Model file for the job. Use its own axes, mm. A direction names the side the tool comes from. Coordinates: 2 decimals unless noted, no trailing zeros. Write each loop counter-clockwise with the first axis right and the second up, starting at its lowest first coordinate (ties: lowest second). Pieces come first, ordered by that corner, then holes. Notation, with made-up numbers: M 44,37 L 66,37 A15 cw 66,60 Z; hole C 60,-19 d7. An arc over 180 degrees is marked long. One line per question, with ' | ' between items. Start each with the question number.
(1) Flat gauge pins, fed straight in: pin 1 Ø1 at (y, z) = (-1.5, -4) entering from -X; pin 2 Ø4 at (y, z) = (4, -33.5) entering from +X; pin 3 Ø11 at (x, y) = (45.5, 7) entering from +Z. Where does each tip first touch, or does it go through?
(2) Cut at A-A (y = 8). Write the cut outline in (x, z).
(3) Cut at D-D (x = 8.5). Write the cut outline in (y, z) (1 decimal), plus the area to 3 significant figures.
(4) Cut at B-B (x = 37). Write the cut outline in (y, z) (1 decimal).
(5) Two-plate mould, pull along X, no slides. Class faces 4 (the face through (1, -1, -8.588)), 5 (the face through (0, 6, -35)), 6 (the face through (42, 6, -35)): +X half, -X half, draft (parallel to the pull), parting line (faces both ways), or undercut.
(6) Tool access for faces 1 (the face through (-5, -1, -28)), 2 (the face through (41, -1, -8.588)), 3 (the face through (47, 10, -6)): list every direction of +Z, -Z, +X, -X, +Y, -Y with a clear straight run to the whole face (end or side of a thin tool).
(7) Cut at C-C (y = 3.75). Write the cut outline in (x, z), plus the area to 3 significant figures.
(8) Wall check: probe 1 along X at (y, z) = (8, -34.65); probe 2 along Z at (x, y) = (48.5, 17); probe 3 along Z at (x, y) = (37, 11). Give the ranges that are in metal, low to high.
from build123d import *

# Parameters (mm, degrees)
SKETCH1_W                    = 42
SKETCH1_H                    = 36
BASE_FLANGE1_DEPTH           = 2
SKETCH6_W                    = 10
SKETCH6_H                    = 24
TAB1_DEPTH                   = 2
SKETCH9_W                    = 10
SKETCH9_H                    = 24
TAB2_DEPTH                   = 2
EDGE_FLANGE1_STRIP_W         = 11.175
EDGE_FLANGE1_STRIP_H         = 2
EDGE_FLANGE1_STRIP_CUT_DEPTH = 42
EDGE_FLANGE1_DEPTH           = 42
EDGE_FLANGE2_START           = -10
EDGE_FLANGE2_DEPTH           = 11
EDGE_FLANGE2_2_DEPTH         = 1
EDGE_FLANGE2_3_DEPTH         = 10
EDGE_FLANGE3_START           = 41
EDGE_FLANGE3_DEPTH           = 11
EDGE_FLANGE3_2_DEPTH         = 1
EDGE_FLANGE3_START_2         = 42
EDGE_FLANGE3_3_DEPTH         = 10
SKETCH21_W                   = 1
SKETCH21_H                   = 4
CUT_EXTRUDE1_DEPTH           = 10
SKETCH22_W                   = 1
SKETCH22_H                   = 4
CUT_EXTRUDE2_DEPTH           = 2
SKETCH23_W                   = 1.5
SKETCH23_H                   = 8.5875
CUT_EXTRUDE3_DEPTH           = 2
SKETCH24_W                   = 1.5
SKETCH24_H                   = 8.5875
CUT_EXTRUDE4_DEPTH           = 2
CUT_EXTRUDE5_REACH           = 67.757
SKETCH26_R                   = 2.5


# Read off the part's stored shape, not the designer's step: Edge-Flange2, Edge-Flange3
# Sheet-metal steps are written as plain solids
with BuildPart() as part:
    # Sketch1 → Base-Flange1 (new body)
    with BuildSketch(Plane(origin=(0, 0, 0), x_dir=(1, 0, 0), z_dir=(0, 1, 0))):
        with Locations((21, 18)):
            Rectangle(SKETCH1_W, SKETCH1_H)
    extrude(amount=-BASE_FLANGE1_DEPTH)

    # Sketch6 → Tab1 (add)
    with BuildSketch(Plane(origin=(0, 0, 0), x_dir=(1, 0, 0), z_dir=(0, 1, 0))):
        with Locations((47, 16)):
            Rectangle(SKETCH6_W, SKETCH6_H)
    extrude(amount=-TAB1_DEPTH)

    # Sketch9 → Tab2 (add)
    with BuildSketch(Plane(origin=(0, 0, 0), x_dir=(1, 0, 0), z_dir=(0, 1, 0))):
        with Locations((-5, 16)):
            Rectangle(SKETCH9_W, SKETCH9_H)
    extrude(amount=-TAB2_DEPTH)

    # Edge-Flange1 strip (across the edge) → Edge-Flange1 strip cut (cut)
    with BuildSketch(Plane(origin=(42, 0, -36), x_dir=(0, 0, 1), z_dir=(-1, 0, 0))):
        with Locations((-2, -1)):
            Rectangle(EDGE_FLANGE1_STRIP_W, EDGE_FLANGE1_STRIP_H)
    extrude(amount=EDGE_FLANGE1_STRIP_CUT_DEPTH, mode=Mode.SUBTRACT)

    # Edge-Flange1 section (across the edge) → Edge-Flange1 (add)
    with BuildSketch(Plane(origin=(42, 0, -36), x_dir=(0, 0, 1), z_dir=(-1, 0, 0))):
        with BuildLine():
            Line((0, 1.5875), (0, 18))
            Line((0, 18), (2, 18))
            Line((2, 18), (2, 1.5875))
            ThreePointArc((2, 1.5875), (2.464967985, 0.464967985), (3.5875, 0))
            Line((3.5875, 0), (3.5875, -2))
            ThreePointArc((3.5875, -2), (1.050754422, -0.949245578), (0, 1.5875))
        make_face()
    extrude(amount=EDGE_FLANGE1_DEPTH)

    # Edge-Flange2 outline → Edge-Flange2 (cut)
    with BuildSketch(Plane.YZ.offset(EDGE_FLANGE2_START)):
        with BuildLine():
            ThreePointArc((-2, -7.5875), (-1.45924519, -5.693430307), (0, -4.370358411))
            Line((0, -4.370358411), (0, -4))
            Line((0, -4), (-2, -4))
            Line((-2, -4), (-2, -7.5875))
        make_face()
    extrude(amount=EDGE_FLANGE2_DEPTH, mode=Mode.SUBTRACT)

    # Edge-Flange2 2 outline → Edge-Flange2 2 (cut)
    with BuildSketch(Plane.YZ):
        with BuildLine():
            Line((0, -8.5875), (0, -4.370358411))
            ThreePointArc((0, -4.370358411), (-1.45924519, -5.693430307), (-2, -7.5875))
            Line((-2, -7.5875), (-2, -8.5875))
            Line((-2, -8.5875), (0, -8.5875))
        make_face()
    extrude(amount=EDGE_FLANGE2_2_DEPTH, mode=Mode.SUBTRACT)

    # Edge-Flange2 3 outline → Edge-Flange2 3 (add)
    with BuildSketch(Plane.YZ.offset(EDGE_FLANGE2_START)):
        with BuildLine():
            Line((18, -4), (1.5875, -4))
            ThreePointArc((1.5875, -4), (0.77243534, -4.093816292), (0, -4.370358411))
            Line((0, -4.370358411), (0, -7.5875))
            ThreePointArc((0, -7.5875), (0.464967985, -6.464967985), (1.5875, -6))
            Line((1.5875, -6), (18, -6))
            Line((18, -6), (18, -4))
        make_face()
    extrude(amount=EDGE_FLANGE2_3_DEPTH)

    # Edge-Flange3 outline → Edge-Flange3 (cut)
    with BuildSketch(Plane.YZ.offset(EDGE_FLANGE3_START)):
        with BuildLine():
            ThreePointArc((-2, -7.5875), (-1.45924519, -5.693430307), (0, -4.370358411))
            Line((0, -4.370358411), (0, -4))
            Line((0, -4), (-2, -4))
            Line((-2, -4), (-2, -7.5875))
        make_face()
    extrude(amount=EDGE_FLANGE3_DEPTH, mode=Mode.SUBTRACT)

    # Edge-Flange3 2 outline → Edge-Flange3 2 (cut)
    with BuildSketch(Plane.YZ.offset(EDGE_FLANGE3_START)):
        with BuildLine():
            Line((0, -8.5875), (0, -4.370358411))
            ThreePointArc((0, -4.370358411), (-1.45924519, -5.693430307), (-2, -7.5875))
            Line((-2, -7.5875), (-2, -8.5875))
            Line((-2, -8.5875), (0, -8.5875))
        make_face()
    extrude(amount=EDGE_FLANGE3_2_DEPTH, mode=Mode.SUBTRACT)

    # Edge-Flange3 3 outline → Edge-Flange3 3 (add)
    with BuildSketch(Plane.YZ.offset(EDGE_FLANGE3_START_2)):
        with BuildLine():
            Line((18, -6), (18, -4))
            Line((18, -4), (1.5875, -4))
            ThreePointArc((1.5875, -4), (0.77243534, -4.093816292), (0, -4.370358411))
            Line((0, -4.370358411), (0, -7.5875))
            ThreePointArc((0, -7.5875), (0.464967985, -6.464967985), (1.5875, -6))
            Line((1.5875, -6), (18, -6))
        make_face()
    extrude(amount=EDGE_FLANGE3_3_DEPTH)

    # Sketch21 → Cut-Extrude1 (cut)
    with BuildSketch(Plane(origin=(0, 0, 0), x_dir=(1, 0, 0), z_dir=(0, 1, 0))):
        with Locations((0.5, 2)):
            Rectangle(SKETCH21_W, SKETCH21_H)
    extrude(amount=-CUT_EXTRUDE1_DEPTH, mode=Mode.SUBTRACT)

    # Sketch22 → Cut-Extrude2 (cut)
    with BuildSketch(Plane(origin=(0, 0, 0), x_dir=(1, 0, 0), z_dir=(0, 1, 0))):
        with Locations((41.5, 2)):
            Rectangle(SKETCH22_W, SKETCH22_H)
    extrude(amount=-CUT_EXTRUDE2_DEPTH, mode=Mode.SUBTRACT)

    # Sketch23 → Cut-Extrude3 (cut)
    with BuildSketch(Plane(origin=(0, 0, 0), x_dir=(1, 0, 0), z_dir=(0, 1, 0))):
        with Locations((1.75, 4.29375)):
            Rectangle(SKETCH23_W, SKETCH23_H)
    extrude(amount=-CUT_EXTRUDE3_DEPTH, mode=Mode.SUBTRACT)

    # Sketch24 → Cut-Extrude4 (cut)
    with BuildSketch(Plane(origin=(0, 0, 0), x_dir=(1, 0, 0), z_dir=(0, 1, 0))):
        with Locations((40.25, 4.29375)):
            Rectangle(SKETCH24_W, SKETCH24_H)
    extrude(amount=-CUT_EXTRUDE4_DEPTH, mode=Mode.SUBTRACT)

    # Sketch26 → Cut-Extrude5 (cut, up to next)
    with BuildSketch(Plane(origin=(0, 0, -36), x_dir=(-1, 0, 0), z_dir=(0, 0, -1)), mode=Mode.PRIVATE) as cut_extrude5_sk1:
        with Locations(Location((-37, 8, 0), (0, 0, 90))):
            Circle(SKETCH26_R)
    cut_extrude5_tool1 = extrude(cut_extrude5_sk1.sketch, amount=-CUT_EXTRUDE5_REACH, mode=Mode.PRIVATE) & part.part
    add(cut_extrude5_tool1.solids().sort_by_distance((37, 8, -36))[0], mode=Mode.SUBTRACT)


solid = part.part
Filled in:
1) pin 1: x = 2.5 | pin 2: x = 42 | pin 3: z = -4
2) outline: M -10,-6 L 0,-6 L 0,-4 L -10,-4 Z; M 0,-36 L 34.5,-36 L 34.5,-34 L 0,-34 Z; M 39.5,-36 L 42,-36 L 42,-34 L 39.5,-34 Z; M 42,-6 L 52,-6 L 52,-4 L 42,-4 Z
3) outline: M -2,-32.4 A3.6 ccw 1.6,-36 L 18,-36 L 18,-34 L 1.6,-34 A1.6 cw 0,-32.4 L 0,0 L -2,0 Z | area: 106 mm²
4) outline: M -2,-32.4 A3.6 ccw 1.6,-36 L 5.5,-36 L 5.5,-34 L 1.6,-34 A1.6 cw 0,-32.4 L 0,0 L -2,0 Z; M 10.5,-36 L 18,-36 L 18,-34 L 10.5,-34 Z
5) face 4: undercut | face 5: -X half | face 6: +X half
6) face 1: -Z, -X, +Y, -Y | face 2: +Z, +Y, -Y | face 3: -Z, +X, -X, +Y
7) outline: M -10,-6 L 0,-6 L 0,-4 L -10,-4 Z; M 0,-36 L 42,-36 L 42,-34 L 0,-34 Z; M 42,-6 L 52,-6 L 52,-4 L 42,-4 Z | area: 124 mm²
8) probe 1: 0 to 34.5, 39.5 to 42 | probe 2: -6 to -4 | probe 3: -36 to -34
